Build history of the part. All positions in model axes, mm. Round coordinates to 2 decimals unless told otherwise and drop trailing zeros. Order: outer loops, then holes, each group sorted by start corner. A loop starts at its lowest first (then second) coordinate and runs counter-clockwise, first axis right, second up. Notation, with made-up numbers: (26.5, 68) -> (43.5, 68) arc R21 ccw to (43.5, 101) -> close; hole circle Ø2 at (83, 25). An arc over 180 degrees is marked (long way). Use a Markdown table: item, result. Add a question column.
Item 1: Slice it at B-B, the plane z = 22.75. Give the cut face in (x, y), plus the area to 3 significant figures.
Item 2: Slice it at A-A, the plane y = -14. Give the cut face in (x, z), plus the area to 3 significant figures.
Item 3: Probe L1, parallel to X at y = -13, z = 25. List the from-to ranges inside material, lowest first.
Item 4: Pin check, flat tip, straight feed: pin 1 (10 mm diameter, centred on y = -11.5, z = 9.5, fed in from -X). Stop position of the tip, or through.
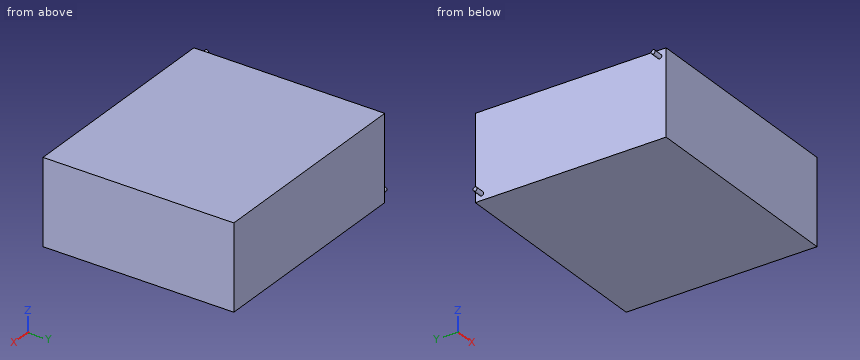
from build123d import *

# Parameters (mm, degrees)
CROQUIS1_W              = 69
CROQUIS1_H              = 60
SALIENTE_EXTRUIR1_DEPTH = 26.7
CROQUIS2_R              = 0.65
SALIENTE_EXTRUIR2_DEPTH = 3


with BuildPart() as part:
    # Croquis1 → Saliente-Extruir1 (new body)
    with BuildSketch(Plane.XY):
        Rectangle(CROQUIS1_W, CROQUIS1_H)
    extrude(amount=SALIENTE_EXTRUIR1_DEPTH)

    # Croquis2 → Saliente-Extruir2 (add)
    with BuildSketch(Plane.ZY.offset(34.5)):
        with Locations((24.7, -28)):
            Circle(CROQUIS2_R)
        with Locations((2, 28)):
            Circle(CROQUIS2_R)
    extrude(amount=SALIENTE_EXTRUIR2_DEPTH)


solid = part.part
Check sheet entries:
| question | item | result |
|---|---|---|
| 1 | outline | (-34.5, -30) -> (34.5, -30) -> (34.5, 30) -> (-34.5, 30) -> close |
| 1 | area | 4,140 mm2 |
| 2 | outline | (-34.5, 0) -> (34.5, 0) -> (34.5, 26.7) -> (-34.5, 26.7) -> close |
| 2 | area | 1,840 mm2 |
| 3 | L1 | -34.5 to 34.5 |
| 4 | pin 1 | x = -34.5 |
